from build123d import *

# Parameters (mm, degrees)
SKETCH_1_W          = 270
SKETCH_1_H          = 20
SKETCH_1_W_2        = 20
SKETCH_1_H_2        = 230
EXTRUDE_1_DEPTH     = 20
CUT_EXTRUDE_1_REACH = 278.089
SKETCH_2_R          = 1.75
CUT_EXTRUDE_2_REACH = 286.825
SKETCH_3_R          = 1.75


with BuildPart() as part:
    # 草图1 → 凸台-拉伸1 (new body)
    with BuildSketch(Plane(origin=(0, 0, 0), x_dir=(1, 0, 0), z_dir=(0, 1, 0))):
        Rectangle(SKETCH_1_W, SKETCH_1_H)
        with Locations((-125, -125)):
            Rectangle(SKETCH_1_W_2, SKETCH_1_H_2)
        with Locations((125, -125)):
            Rectangle(SKETCH_1_W_2, SKETCH_1_H_2)
    extrude(amount=EXTRUDE_1_DEPTH)

    # 草图2 → 切除-拉伸1 (cut, up to next)
    with BuildSketch(Plane(origin=(0, 20, 0), x_dir=(1, 0, 0), z_dir=(0, 1, 0)), mode=Mode.PRIVATE) as cut_extrude_1_sk1:
        with Locations(Location((-125, 0, 0), (0, 0, 270))):
            Circle(SKETCH_2_R)
    cut_extrude_1_tool1 = extrude(cut_extrude_1_sk1.sketch, amount=-CUT_EXTRUDE_1_REACH, mode=Mode.PRIVATE) & part.part
    # 草图2 → 切除-拉伸1 (cut, up to next)
    with BuildSketch(Plane(origin=(0, 20, 0), x_dir=(1, 0, 0), z_dir=(0, 1, 0)), mode=Mode.PRIVATE) as cut_extrude_1_sk2:
        with Locations(Location((-125, -20, 0), (0, 0, 270))):
            Circle(SKETCH_2_R)
    cut_extrude_1_tool2 = extrude(cut_extrude_1_sk2.sketch, amount=-CUT_EXTRUDE_1_REACH, mode=Mode.PRIVATE) & part.part
    # 草图2 → 切除-拉伸1 (cut, up to next)
    with BuildSketch(Plane(origin=(0, 20, 0), x_dir=(1, 0, 0), z_dir=(0, 1, 0)), mode=Mode.PRIVATE) as cut_extrude_1_sk3:
        with Locations(Location((-105, 0, 0), (0, 0, 270))):
            Circle(SKETCH_2_R)
    cut_extrude_1_tool3 = extrude(cut_extrude_1_sk3.sketch, amount=-CUT_EXTRUDE_1_REACH, mode=Mode.PRIVATE) & part.part
    # 草图2 → 切除-拉伸1 (cut, up to next)
    with BuildSketch(Plane(origin=(0, 20, 0), x_dir=(1, 0, 0), z_dir=(0, 1, 0)), mode=Mode.PRIVATE) as cut_extrude_1_sk4:
        with Locations(Location((-125, -210, 0), (0, 0, 270))):
            Circle(SKETCH_2_R)
    cut_extrude_1_tool4 = extrude(cut_extrude_1_sk4.sketch, amount=-CUT_EXTRUDE_1_REACH, mode=Mode.PRIVATE) & part.part
    # 草图2 → 切除-拉伸1 (cut, up to next)
    with BuildSketch(Plane(origin=(0, 20, 0), x_dir=(1, 0, 0), z_dir=(0, 1, 0)), mode=Mode.PRIVATE) as cut_extrude_1_sk5:
        with Locations(Location((-125, -230, 0), (0, 0, 270))):
            Circle(SKETCH_2_R)
    cut_extrude_1_tool5 = extrude(cut_extrude_1_sk5.sketch, amount=-CUT_EXTRUDE_1_REACH, mode=Mode.PRIVATE) & part.part
    # 草图2 → 切除-拉伸1 (cut, up to next)
    with BuildSketch(Plane(origin=(0, 20, 0), x_dir=(1, 0, 0), z_dir=(0, 1, 0)), mode=Mode.PRIVATE) as cut_extrude_1_sk6:
        with Locations(Location((125, -210, 0), (0, 0, 270))):
            Circle(SKETCH_2_R)
    cut_extrude_1_tool6 = extrude(cut_extrude_1_sk6.sketch, amount=-CUT_EXTRUDE_1_REACH, mode=Mode.PRIVATE) & part.part
    # 草图2 → 切除-拉伸1 (cut, up to next)
    with BuildSketch(Plane(origin=(0, 20, 0), x_dir=(1, 0, 0), z_dir=(0, 1, 0)), mode=Mode.PRIVATE) as cut_extrude_1_sk7:
        with Locations(Location((125, -230, 0), (0, 0, 270))):
            Circle(SKETCH_2_R)
    cut_extrude_1_tool7 = extrude(cut_extrude_1_sk7.sketch, amount=-CUT_EXTRUDE_1_REACH, mode=Mode.PRIVATE) & part.part
    # 草图2 → 切除-拉伸1 (cut, up to next)
    with BuildSketch(Plane(origin=(0, 20, 0), x_dir=(1, 0, 0), z_dir=(0, 1, 0)), mode=Mode.PRIVATE) as cut_extrude_1_sk8:
        with Locations(Location((125, 0, 0), (0, 0, 270))):
            Circle(SKETCH_2_R)
    cut_extrude_1_tool8 = extrude(cut_extrude_1_sk8.sketch, amount=-CUT_EXTRUDE_1_REACH, mode=Mode.PRIVATE) & part.part
    # 草图2 → 切除-拉伸1 (cut, up to next)
    with BuildSketch(Plane(origin=(0, 20, 0), x_dir=(1, 0, 0), z_dir=(0, 1, 0)), mode=Mode.PRIVATE) as cut_extrude_1_sk9:
        with Locations(Location((125, -20, 0), (0, 0, 270))):
            Circle(SKETCH_2_R)
    cut_extrude_1_tool9 = extrude(cut_extrude_1_sk9.sketch, amount=-CUT_EXTRUDE_1_REACH, mode=Mode.PRIVATE) & part.part
    # 草图2 → 切除-拉伸1 (cut, up to next)
    with BuildSketch(Plane(origin=(0, 20, 0), x_dir=(1, 0, 0), z_dir=(0, 1, 0)), mode=Mode.PRIVATE) as cut_extrude_1_sk10:
        with Locations(Location((105, 0, 0), (0, 0, 270))):
            Circle(SKETCH_2_R)
    cut_extrude_1_tool10 = extrude(cut_extrude_1_sk10.sketch, amount=-CUT_EXTRUDE_1_REACH, mode=Mode.PRIVATE) & part.part
    # 草图2 → 切除-拉伸1 (cut, up to next)
    with BuildSketch(Plane(origin=(0, 20, 0), x_dir=(1, 0, 0), z_dir=(0, 1, 0)), mode=Mode.PRIVATE) as cut_extrude_1_sk11:
        with Locations(Location((85, 0, 0), (0, 0, 270))):
            Circle(SKETCH_2_R)
    cut_extrude_1_tool11 = extrude(cut_extrude_1_sk11.sketch, amount=-CUT_EXTRUDE_1_REACH, mode=Mode.PRIVATE) & part.part
    # 草图2 → 切除-拉伸1 (cut, up to next)
    with BuildSketch(Plane(origin=(0, 20, 0), x_dir=(1, 0, 0), z_dir=(0, 1, 0)), mode=Mode.PRIVATE) as cut_extrude_1_sk12:
        with Locations(Location((-85, 0, 0), (0, 0, 270))):
            Circle(SKETCH_2_R)
    cut_extrude_1_tool12 = extrude(cut_extrude_1_sk12.sketch, amount=-CUT_EXTRUDE_1_REACH, mode=Mode.PRIVATE) & part.part
    add(cut_extrude_1_tool1.solids().sort_by_distance((-125, 20, 0))[0], mode=Mode.SUBTRACT)
    add(cut_extrude_1_tool2.solids().sort_by_distance((-125, 20, 20))[0], mode=Mode.SUBTRACT)
    add(cut_extrude_1_tool3.solids().sort_by_distance((-105, 20, 0))[0], mode=Mode.SUBTRACT)
    add(cut_extrude_1_tool4.solids().sort_by_distance((-125, 20, 210))[0], mode=Mode.SUBTRACT)
    add(cut_extrude_1_tool5.solids().sort_by_distance((-125, 20, 230))[0], mode=Mode.SUBTRACT)
    add(cut_extrude_1_tool6.solids().sort_by_distance((125, 20, 210))[0], mode=Mode.SUBTRACT)
    add(cut_extrude_1_tool7.solids().sort_by_distance((125, 20, 230))[0], mode=Mode.SUBTRACT)
    add(cut_extrude_1_tool8.solids().sort_by_distance((125, 20, 0))[0], mode=Mode.SUBTRACT)
    add(cut_extrude_1_tool9.solids().sort_by_distance((125, 20, 20))[0], mode=Mode.SUBTRACT)
    add(cut_extrude_1_tool10.solids().sort_by_distance((105, 20, 0))[0], mode=Mode.SUBTRACT)
    add(cut_extrude_1_tool11.solids().sort_by_distance((85, 20, 0))[0], mode=Mode.SUBTRACT)
    add(cut_extrude_1_tool12.solids().sort_by_distance((-85, 20, 0))[0], mode=Mode.SUBTRACT)

    # 草图3 → 切除-拉伸2 (cut, up to next)
    with BuildSketch(Plane(origin=(0, 0, -10), x_dir=(-1, 0, 0), z_dir=(0, 0, -1)), mode=Mode.PRIVATE) as cut_extrude_2_sk1:
        with Locations((-20, 10)):
            Circle(SKETCH_3_R)
    cut_extrude_2_tool1 = extrude(cut_extrude_2_sk1.sketch, amount=-CUT_EXTRUDE_2_REACH, mode=Mode.PRIVATE) & part.part
    # 草图3 → 切除-拉伸2 (cut, up to next)
    with BuildSketch(Plane(origin=(0, 0, -10), x_dir=(-1, 0, 0), z_dir=(0, 0, -1)), mode=Mode.PRIVATE) as cut_extrude_2_sk2:
        with Locations((0, 10)):
            Circle(SKETCH_3_R)
    cut_extrude_2_tool2 = extrude(cut_extrude_2_sk2.sketch, amount=-CUT_EXTRUDE_2_REACH, mode=Mode.PRIVATE) & part.part
    # 草图3 → 切除-拉伸2 (cut, up to next)
    with BuildSketch(Plane(origin=(0, 0, -10), x_dir=(-1, 0, 0), z_dir=(0, 0, -1)), mode=Mode.PRIVATE) as cut_extrude_2_sk3:
        with Locations((-40, 10)):
            Circle(SKETCH_3_R)
    cut_extrude_2_tool3 = extrude(cut_extrude_2_sk3.sketch, amount=-CUT_EXTRUDE_2_REACH, mode=Mode.PRIVATE) & part.part
    add(cut_extrude_2_tool1.solids().sort_by_distance((20, 10, -10))[0], mode=Mode.SUBTRACT)
    add(cut_extrude_2_tool2.solids().sort_by_distance((0, 10, -10))[0], mode=Mode.SUBTRACT)
    add(cut_extrude_2_tool3.solids().sort_by_distance((40, 10, -10))[0], mode=Mode.SUBTRACT)


solid = part.part
Geometry: final body of the model. Coordinates: model frame, mm. A direction names the side the tool comes from. Coordinates: 2 decimals unless noted, no trailing zeros. Loops run counter-clockwise (first coordinate to the right, second up) from the corner with the lowest first, then second, coordinate; pieces in that order, holes last. Notation, with made-up numbers: (-35, 72) - (8, 72) arc R9 ccw to (8, 76) - close; hole circle Ø2 at (-25, 18.25). An arc over 180 degrees is marked (long way). Put each result on its own line as item: value. Start each with the question number.
Q1. Pull-direction query (X, two-part tool) for faces 3 (the flat face through (-135, 10, 113)), 4 (the flat face through (115, 10, 127)), 5 (the flat face through (-125, 10, 240)), 6 (the flat face through (135, 10, 117)); classes: released by +X, released by -X, zero draft, split by the parting line, or undercut.
Q2. Line query: line 1 (Z direction, x = -125, y = 14); line 2 (X direction, y = 11, z = 210); line 3 (X direction, y = 15, z = 143.5). Output: solid intervals per line, ascending.
Q3. Pin query (flat end, axial travel): pin 1 Ø1 at (x, y) = (-102.5, 8.5) entering from +Z. Return the tip coordinate at first contact, or that it passes through.
Q4. Cut plane A-A, the plane y = 16.75. Give the number of separate pieces and of enclosed holes in the cut face, and give its area (3 significant figures).
Q5. Cut plane B-B, the plane x = -63.5. Return loops of the section in (y, z), and give its area (3 significant figures).
Q6. Set-up query: faces 1 (the flat face through (-2, 12, 10)), 2 (the flat face through (125, 10, 240)). Return all of +Z, -Z, +X, -X, +Y, -Y with unobstructed straight access to the full face (end or side cutting, diameter ignored); none if empty.
Filled sheet:
1. face 3: released by -X
1. face 4: undercut
1. face 5: zero draft
1. face 6: released by +X
2. line 1: -10 to -1.75, 1.75 to 18.25, 21.75 to 208.25, 211.75 to 228.25, 231.75 to 240
2. line 2: -135 to -126.75, -123.25 to -115, 115 to 123.25, 126.75 to 135
2. line 3: -135 to -115, 115 to 135
3. pin 1: z = 10
4. separate pieces: 1
4. enclosed holes: 12
4. area: 14,500 mm²
5. outline: (0, -10) - (20, -10) - (20, 10) - (0, 10) - close
5. area: 400 mm²
6. face 1: +Z, +Y, -Y
6. face 2: +Z, +X, -X, +Y, -Y
